Here's how the part is built. I have some questions about the finished solid (model axes, mm). A direction names the side the tool comes from. Round coordinates to 2 decimals unless told otherwise and drop trailing zeros. Loops run counter-clockwise (first coordinate to the right, second up) from the corner with the lowest first, then second, coordinate; pieces in that order, holes last. Notation, with made-up numbers: M 64.25,-13.75 L 95.25,-13.75 A28 ccw 95.25,4.25 Z; hole C 41,69.5 d7. An arc over 180 degrees is marked long. Use a Markdown table: item, result.
from build123d import *

# Parameters (mm, degrees)
SKETCH_1_W      = 85
SKETCH_1_H      = 12
EXTRUDE_1_DEPTH = 43
SKETCH_3_W      = 6
SKETCH_3_H      = 42
EXTRUDE_3_DEPTH = 18
FILLET_1_R      = 5
FILLET_2_R      = 2


with BuildPart() as part:
    # 草圖1 → 伸長1 (new, symmetric)
    with BuildSketch(Plane.XY):
        with Locations((42.5, -48)):
            Rectangle(SKETCH_1_W, SKETCH_1_H)
    extrude(amount=EXTRUDE_1_DEPTH, both=True)

    # 草圖3 → 伸長3 (add, symmetric)
    with BuildSketch(Plane.XY):
        with Locations((82, -21)):
            Rectangle(SKETCH_3_W, SKETCH_3_H)
    extrude(amount=EXTRUDE_3_DEPTH, both=True)

    # 圓角1
    fillet_1_edges = [part.edges().sort_by_distance(p)[0] for p in [
        (85, -48, -43),
        (85, -48, 43),
    ]]
    fillet(fillet_1_edges, radius=FILLET_1_R)

    # 圓角2
    fillet_2_edges = [part.edges().sort_by_distance(p)[0] for p in [
        (85, -42, -28),
        (82, -42, -18),
        (79, -42, 0),
        (85, -21, -18),
        (79, -21, -18),
        (82, -42, 18),
        (85, -21, 18),
        (79, -21, 18),
        (85, -42, 28),
        (40, -42, -43),
        (40, -42, 43),
        (83.535533906, -42, 41.535533906),
        (83.535533906, -42, -41.535533906),
    ]]
    fillet(fillet_2_edges, radius=FILLET_2_R)


solid = part.part
1. We'd pull the mould along X, two halves only. Please class faces 6 (the face through (82.01, -41.43, 18.6)), 7 (the face through (83, -49, -42)), 8 (the face through (79.6, -19.72, 17.43)): +X half, -X half, draft (parallel to the pull), parting line (faces both ways), or undercut.
Answer sheet:
| item | result |
|---|---|
| face 6 | draft |
| face 7 | +X half |
| face 8 | -X half |
2. Imagine slicing it at A-A, the plane y = -32. Write out the boundary of the cut face in (x, z).
Answer sheet:
| item | result |
|---|---|
| outline | M 79,-16 A2 ccw 81,-18 L 83,-18 A2 ccw 85,-16 L 85,16 A2 ccw 83,18 L 81,18 A2 ccw 79,16 Z |
3. Which directions (+Z, -Z, +X, -X, +Y, -Y) give clear straight access to the entire face, cutting with the end or side of a thin tool? Please do faces 1 (the face through (84.43, -42.6, -29.13)), 2 (the face through (79, -20, 0)), 3 (the face through (82, -20, -18)), 4 (the face through (84.43, -19.72, 17.4)), 5 (the face through (82, -20, 18)).
Answer sheet:
| item | result |
|---|---|
| face 1 | -Z, +X, +Y |
| face 2 | +Z, -Z, -X, +Y |
| face 3 | -Z, +X, -X, +Y |
| face 4 | +Z, +X, +Y |
| face 5 | +Z, +X, -X, +Y |
4. Imagine slicing it at D-D, the plane z = -32.5. Write out the boundary of the cut face in (x, y), then the cut area to 3 significant figures.
Answer sheet:
| item | result |
|---|---|
| outline | M 0,-54 L 85,-54 L 85,-44 A2 ccw 83,-42 L 0,-42 Z |
| area | 1,020 mm2 |
5. I need wall thicknesses on probe 1 along X at (y, z) = (-28, -3); probe 2 along Y at (x, z) = (26.5, 35.5). Which ranges of each line are inside material? Lowest first, please. Write a range as from..to.
Answer sheet:
| item | result |
|---|---|
| probe 1 | 79..85 |
| probe 2 | -54..-42 |
6. For pin 1 Ø12 at (x, z) = (46.5, -6) entering from +Y; pin 2 Ø1.5 at (y, z) = (-13.5, 16) entering from -X; pin 3 Ø0.6 at (x, y) = (82, -15) entering from +Z, each with a flat end and sliding along its axis, tell me the tip position at first contact or that it passes through.
Answer sheet:
| item | result |
|---|---|
| pin 1 | y = -42 |
| pin 2 | x = 79 |
| pin 3 | z = 18 |
7. Imagine slicing it at C-C, the plane x = 70. Write out the boundary of the cut face in (y, z).
Answer sheet:
| item | result |
|---|---|
| outline | M -54,-43 L -44,-43 A2 ccw -42,-41 L -42,41 A2 ccw -44,43 L -54,43 Z |
8. Imagine slicing it at B-B, the plane z = 13.5. Write out the boundary of the cut face in (x, y).
Answer sheet:
| item | result |
|---|---|
| outline | M 0,-54 L 85,-54 L 85,0 L 79,0 L 79,-40 A2 cw 77,-42 L 0,-42 Z |
